For this review, take the finished solid that the model builds, in its own axes (mm). A direction names the side the tool comes from. Give positions to 0.01 mm unless a question says otherwise; leave off trailing zeros. Order: outer loops, then holes, each group sorted by start corner. A loop starts at its lowest first (then second) coordinate and runs counter-clockwise, first axis right, second up. Notation, with made-up numbers: M -22.5,-9 L 6.5,-9 A21 ccw 6.5,23 Z; hole C 82.5,26.5 d1. An arc over 180 degrees is marked long. Answer as CSV lines item,"result". Start each with the question number.
1. For line 1 along X through (y, z) = (1, 3.25); line 2 along X through (y, z) = (0.5, 3.65); line 3 along Y through (x, z) = (0.4, 0.55), list the stretches that pass through material, from the lowest coordinate up.
2. We need section A-A, the plane z = 0.7. Give the boundary of the cut face in (x, y).
3. Clearance check with flat-ended pins moving along their axes: P1, Ø1.1, axis at x = 2.5, y = -1.5, coming from the +Z side; P2, Ø0.7, axis at x = 2.5, y = 1.5, coming from the +Z side; P3, Ø0.7, axis at x = -2, y = 1.5, coming from the +Z side. State where each tip first meets the part, or that it passes through.
4. Mouldability with a two-part tool opening along X and no side actions: class faces 1 (the flat face through (1, -1, 4)), 2 (the cylindrical face through (-0.27, -1.22, 2.03)), 3 (the flat face through (1.37, 2.41, 1.48)) as pulls with the +X half, pulls with the -X half, needs draft (parallel to the pull), parting line crosses it, or undercut.
5. We need section B-B, the plane z = 3.4. Give the boundary of the cut face in (x, y), and give its area (3 significant figures).
6. Machinability: for faces 4 (the flat face through (2.54, -1.46, 3)), 5 (the flat face through (-2.54, 1.47, 3)), 6 (the flat face through (2.54, 1.47, 3)), 7 (the flat face through (-2.54, -1.46, 3)), 8 (the flat face through (-1.37, -2.41, 1.48)), which of the approach directions +Z, -Z, +X, -X, +Y, -Y give a long, thin tool a straight path to every point of the face, cutting with its end or side? Answer none if there is none.
Autodesk Inventor part; units mm, degrees
ref_plane "YZ Plane" through (0, 0, 0) normal (1, 0, 0) x (0, 1, 0)
ref_plane "XZ Plane" through (0, 0, 0) normal (0, 1, 0) x (-1, 0, 0)
ref_plane "XY Plane" through (0, 0, 0) normal (0, 0, 1) x (1, 0, 0)
sketch "スケッチ1" plane through (0, 0, 0) normal (0, 0, 1) x (1, 0, 0)
  line L0 (0, -3.2) -> (-2.7713, -1.6)
  line L1 (-2.7713, -1.6) -> (-2.7713, 1.6)
  line L2 (-2.7713, 1.6) -> (0, 3.2)
  line L3 (0, 3.2) -> (2.7713, 1.6)
  line L4 (2.7713, 1.6) -> (2.7713, -1.6)
  line L5 (2.7713, -1.6) -> (0, -3.2)
  circle A0 centre (0, 0) radius 2.7713
  dimension "d0" = 6.4
extrude "押し出し1" add sketch "スケッチ1" along normal blind 3
sketch "スケッチ2" plane through (0, 0, 3) normal (0, 0, 1) x (1, 0, 0)
  line L0 (-2.7713, -1.6) -> (0, -3.2)
  line L1 (0, -3.2) -> (2.7713, -1.6)
  line L2 (2.7713, -1.6) -> (2.7713, 1.6)
  line L3 (2.7713, 1.6) -> (0, 3.2)
  line L4 (0, 3.2) -> (-2.7713, 1.6)
  line L5 (-2.7713, 1.6) -> (-2.7713, -1.6)
  circle A0 centre (0, 0) radius 2.7713
extrude "押し出し2" add sketch "スケッチ2" along normal blind 1 contours A0
chamfer "面取り1" distance 1 angle 45 1 edges at (-2.7713, 0, 4)
sketch "スケッチ3" plane through (0, 0, 4) normal (0, 0, 1) x (1, 0, 0)
  circle A0 centre (0, 0) radius 1.7713
  circle A1 centre (0, 0) radius 1.25
  dimension "d8" = 2.5
extrude "押し出し3" cut sketch "スケッチ3" against normal blind 4 contours A1
thread "ねじ1"
properties part number "ナイロンナット" material "アルミニウム"
Result set:
1,line 1,"-2.32 to -0.75, 0.75 to 2.32"
1,line 2,"-2.06 to -1.15, 1.15 to 2.06"
1,line 3,"-2.97 to -1.18, 1.18 to 2.97"
2,outline,"M -2.77,-1.6 L 0,-3.2 L 2.77,-1.6 L 2.77,1.6 L 0,3.2 L -2.77,1.6 Z; hole C 0,0 d2.5"
3,P1,"z = 3.41"
3,P2,"z = 3.21"
3,P3,"z = 3.62"
4,face 1,"needs draft"
4,face 2,"undercut"
4,face 3,"pulls with the +X half"
5,outline,"C 0,0 d4.74; hole C 0,0 d2.5"
5,area,"12.8 mm2"
6,face 4,"+Z, +X, -Y"
6,face 5,"+Z, -X, +Y"
6,face 6,"+Z, +X, +Y"
6,face 7,"+Z, -X, -Y"
6,face 8,"+Z, -Z, -X, -Y"
